Geometry: see drawing. Coordinates: mm, zero at the bounding-box minimum. Give positions to 0.01 mm unless a question says otherwise; leave off trailing zeros. Order: outer loops, then holes, each group sorted by start corner. A loop starts at its lowest first (then second) coordinate and runs counter-clockwise, first axis right, second up. Notation, with made-up numbers: M 49.25,64 L 101.25,64 A11 ccw 101.25,85 Z; hole C 37.5,15.25 d9. An arc over 180 degrees is marked long. Use a Markdown table: item, result.
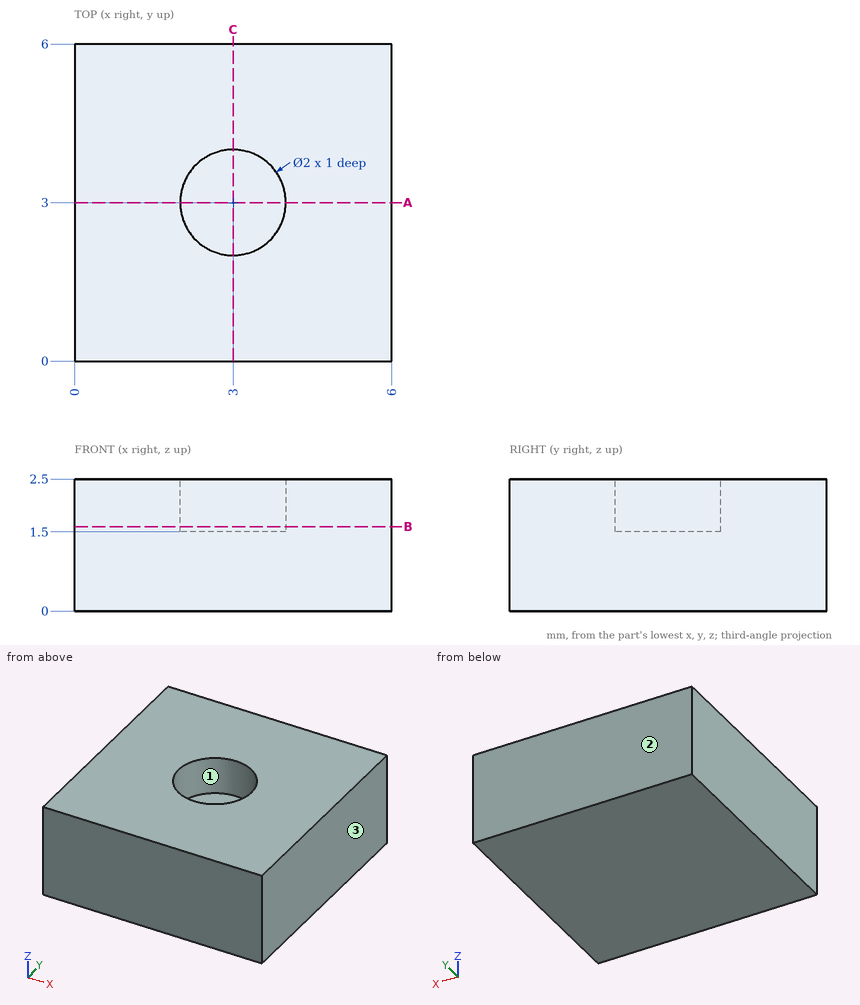
1) Material intervals for line 1 (Y direction, x = 3, z = 1.7); line 2 (Z direction, x = 3.6, y = 2.3); line 3 (Y direction, x = 3.7, z = 2.1), sorted ascending. Write a range as from..to.
Response values:
| item | result |
|---|---|
| line 1 | y = 0..2, 4..6 |
| line 2 | z = 0..1.5 |
| line 3 | y = 0..2.29, 3.71..6 |
2) Mould query, pull axis X, two halves, no side actions, for the marked faces 1, 2 and 3. Classes: released by +X, released by -X, zero draft, split by the parting line, or undercut.
Response values:
| item | result |
|---|---|
| face 1 | undercut |
| face 2 | zero draft |
| face 3 | released by +X |
3) Cut plane B-B on z = 1.6. Return loops of the section in (x, y), and give its area (3 significant figures).
Response values:
| item | result |
|---|---|
| outline | M 0,0 L 6,0 L 6,6 L 0,6 Z; hole C 3,3 d2 |
| area | 32.9 mm² |
4) Cut plane A-A on y = 3. Return loops of the section in (x, z), and give its area (3 significant figures).
Response values:
| item | result |
|---|---|
| outline | M 0,0 L 6,0 L 6,2.5 L 4,2.5 L 4,1.5 L 2,1.5 L 2,2.5 L 0,2.5 Z |
| area | 13.0 mm² |
5) First-contact query: pin 1 Ø1.6 at (x, y) = (3, 3) entering from -Z. Flat tip, straight axial feed; report the tip coordinate or a pass-through.
Response values:
| item | result |
|---|---|
| pin 1 | stops at z = 0 |
